Here's how the part is built. I have some questions about the finished solid (model axes, mm). Coordinates: 2 decimals unless noted, no trailing zeros. Write each loop counter-clockwise with the first axis right and the second up, starting at its lowest first coordinate (ties: lowest second). Pieces come first, ordered by that corner, then holes.
```python
from build123d import *

# Parameters (mm, degrees)
F0_W        = 38.1
F0_H        = 38.1
F1_DEPTH    = 4.699
F2_R        = 2.54
F3_T1_DEPTH = 50.6563121576
F4_T1_DEPTH = 48.26
F5_T1_DEPTH = 48.1450497261


# Not quite as in the source:
# - a fillet or chamfer that OpenCascade refuses, or shapes differently, is made with other operations: its cross-section is extruded or revolved along the edge and cut away or added


with BuildPart() as f1:
    # F0 (on Front) → F1 (new body)
    with BuildSketch(Plane.XZ):
        Rectangle(F0_W, F0_H)
    extrude(amount=F1_DEPTH)

    # F2
    f2_edges = [f1.edges().sort_by_distance(p)[0] for p in [
        (19.05, -4.699, 0),
    ]]
    fillet(f2_edges, radius=F2_R)

    # F3: fillet of radius 2.54 on 1 edges, made by hand

    # F3_s2 → F3_t1 (cut)
    with BuildSketch(Plane.XY.offset(-25.3281560788)):
        with BuildLine():
            ThreePointArc((19.05, -2.159), (18.1946149794, -0.6139496372), (16.5387375685, 0))
            Line((16.5387375685, 0), (19.05, 0))
            Line((19.05, 0), (19.05, -2.159))
        make_face()
    extrude(amount=F3_T1_DEPTH, mode=Mode.SUBTRACT)

    # F4: fillet of radius 2.54 on 1 edges, made by hand

    # F4_s2 → F4_t1 (cut)
    with BuildSketch(Plane.YZ.offset(-25.4)):
        with BuildLine():
            ThreePointArc((-2.159, 19.05), (-3.9550512242, 18.3060512242), (-4.699, 16.51))
            Line((-4.699, 16.51), (-4.699, 19.05))
            Line((-4.699, 19.05), (-2.159, 19.05))
        make_face()
    extrude(amount=F4_T1_DEPTH, mode=Mode.SUBTRACT)

    # F5: fillet of radius 2.54 on 1 edges, made by hand

    # F5_s2 → F5_t1 (cut)
    with BuildSketch(Plane.YZ.offset(-25.3281560788)):
        with BuildLine():
            ThreePointArc((-2.159, 19.05), (-0.6139496372, 18.1946149794), (0, 16.5387375685))
            Line((0, 16.5387375685), (0, 19.05))
            Line((0, 19.05), (-2.159, 19.05))
        make_face()
    extrude(amount=F5_T1_DEPTH, mode=Mode.SUBTRACT)


solid = f1.part
```
1) Imagine slicing it at A-A on x = 10. Please give me the cut outline in (y, z).
Values follow:
outline: (-4.7, -19.05) - (0, -19.05) - (0, 16.54) arc R2.54 ccw to (-2.16, 19.05) arc R2.54 ccw to (-4.7, 16.51) - close
2) I need wall thicknesses on probe 1 along Z at (x, y) = (6.5, -4.25); probe 2 along X at (y, z) = (-3.8, -3); probe 3 along X at (y, z) = (-1, -8). Which ranges of each line are inside material? Lowest first, please.
Values follow:
probe 1: z = -19.05 to 17.95
probe 2: x = -19.05 to 18.45
probe 3: x = -19.05 to 18.56
3) Will these pins go through, and if not, where does the flat tip stop? pin 1 (1.5 mm diameter, centred on y = -0.5, z = 7.5, fed in from +X); pin 2 (2 mm diameter, centred on y = -1, z = 9.5, fed in from +X).
Values follow:
pin 1: stops at x = 18.73
pin 2: stops at x = 19.02
4) Imagine slicing it at B-B on z = 5. Please give me the cut outline in (x, y).
Values follow:
outline: (-19.05, -4.7) - (16.51, -4.7) arc R2.54 ccw to (19.05, -2.16) arc R2.54 ccw to (16.54, 0) - (-19.05, 0) - close
